Autodesk Inventor part; units mm, degrees
ref_plane "YZ Plane" through (0, 0, 0) normal (1, 0, 0) x (0, 1, 0)
ref_plane "XZ Plane" through (0, 0, 0) normal (0, 1, 0) x (-1, 0, 0)
ref_plane "XY Plane" through (0, 0, 0) normal (0, 0, 1) x (1, 0, 0)
sketch "Sketch1" plane through (0, 0, 0) normal (0, 1, 0) x (-1, 0, 0)
  line L0 (40, 37.5) -> (-40, 37.5)
  line L1 (-40, 37.5) -> (-40, -37.5)
  line L2 (-40, -37.5) -> (40, -37.5)
  line L3 (40, -37.5) -> (40, 37.5)
  line L4 (40, 37.5) -> (-40, -37.5) construction
  line L5 (-40, 37.5) -> (40, -37.5) construction
  point P0 (0, 0)
  dimension "d0" = 80
  dimension "d1" = 75
extrude "Extrusion1" add sketch "Sketch1" along normal blind 3
sketch "Sketch2" plane through (0, 0, 0) normal (0, -1, 0) x (1, 0, 0)
  line L0 (-38, -35.5) -> (38, -35.5)
  line L1 (38, -35.5) -> (38, 35.5)
  line L2 (38, 35.5) -> (-38, 35.5)
  line L3 (-38, 35.5) -> (-38, -35.5)
  line L4 (-38, -35.5) -> (38, 35.5) construction
  line L5 (38, -35.5) -> (-38, 35.5) construction
  line L6 (-40, -37.5) -> (-40, 37.5)
  line L7 (-40, 37.5) -> (40, 37.5)
  line L8 (-40, -37.5) -> (40, -37.5)
  line L9 (40, -37.5) -> (40, 37.5)
  line L10 (40, 37.5) -> (-40, 37.5)
  line L11 (-40, 37.5) -> (-40, -37.5)
  line L12 (-40, -37.5) -> (40, 37.5) construction
  line L13 (40, -37.5) -> (-40, 37.5) construction
  point P0 (0, 0)
  dimension "d4" = 2
  dimension "d5" = 2
extrude "Extrusion2" add sketch "Sketch2" along normal blind 30
sketch "Sketch3" plane through (40, 3, 37.5) normal (1, 0, 0) x (0, 0, -1)
  line L0 (73, -33) -> (2, -33)
  line L1 (12.5, -33) -> (62.5, -33)
  line L2 (62.5, -33) -> (62.5, -24)
  line L3 (62.5, -24) -> (12.5, -24)
  line L4 (12.5, -24) -> (12.5, -33)
  line L5 (75, -33) -> (75, 0)
  point P0 (37.5, -3)
  dimension "d8" = 50
  dimension "d9" = 9
  dimension "d10" = 12.5
extrude "Extrusion3" cut sketch "Sketch3" against normal up to surface (2 mm away)
sketch "Sketch4" plane through (-40, 3, 37.5) normal (0, 0, 1) x (1, 0, 0)
  line L0 (78, -33) -> (2, -33)
  line L1 (2, -33) -> (22, -33)
  line L2 (22, -33) -> (22, -13)
  line L3 (22, -13) -> (2, -13)
  line L4 (2, -13) -> (2, -33)
  line L5 (0, -33) -> (0, 0)
  line L6 (22, -33) -> (28, -33)
  line L7 (28, -33) -> (28, -27)
  line L8 (28, -27) -> (22, -27)
  line L9 (22, -27) -> (22, -33)
  point P0 (40, -3)
  point P1 (22, -27)
  dimension "d13" = 20
  dimension "d14" = 20
  dimension "d15" = 2
  dimension "d16" = 6
  dimension "d17" = 6
extrude "Extrusion4" cut sketch "Sketch4" against normal up to surface (2 mm away)
fillet "Fillet1" radius 2 4 edges at (-38, -10, 36.5) (-18, -10, 36.5) (-12, -24, 36.5) (-18, -24, 36.5)
fillet "Fillet2" radius 2 2 edges at (39, -21, 25) (39, -21, -25)
sketch "Sketch5" plane through (40, 3, -37.5) normal (0, 0, -1) x (-1, 0, 0)
  line L0 (2, -33) -> (78, -33)
  line L1 (78, -33) -> (63, -33)
  line L2 (63, -33) -> (63, -23)
  line L3 (63, -23) -> (78, -23)
  line L4 (78, -23) -> (78, -33)
  line L5 (80, -33) -> (80, 0)
  point P0 (40, -3)
  point P1 (78, -28)
  dimension "d22" = 15
  dimension "d23" = 10
  dimension "d24" = 2
extrude "Extrusion5" cut sketch "Sketch5" against normal up to surface (2 mm away)
fillet "Fillet3" radius 2 3 edges at (-38, -20, -36.5) (-23, -20, -36.5) (-23, -30, -36.5)
sketch "Sketch6" plane through (40, 3, -37.5) normal (0, 0, -1) x (-1, 0, 0)
  circle A0 centre (27, -28) radius 2.25
  line L0 (61, -33) -> (0, -33)
  line L1 (0, -33) -> (0, 0)
  point P0 (40, -3)
  dimension "d28" = 4.5
  dimension "d29" = 5
  dimension "d30" = 27
extrude "Extrusion6" cut sketch "Sketch6" against normal through all
sketch "Sketch7" plane through (-40, 3, -37.5) normal (-1, 0, 0) x (0, 0, 1)
  circle A0 centre (37.5, -28) radius 2.25
  line L0 (75, -33) -> (0, -33)
  line L1 (75, -33) -> (75, 0)
  point P0 (37.5, -3)
  dimension "d33" = 4.5
  dimension "d34" = 5
  dimension "d35" = 37.5
extrude "Extrusion7" cut sketch "Sketch7" against normal up to surface (2 mm away)
fillet "Fillet4" radius 5 4 edges at (-40, 3, 0) (0, 3, 37.5) (0, 3, -37.5) (40, 3, 0)
fillet "Fillet5" radius 5 8 edges at (38.5355, 1.5355, -36.0355) (40, -16, -37.5) (-38.5355, 1.5355, -36.0355) (-40, -16, -37.5) (-38.5355, 1.5355, 36.0355) (-40, -16, 37.5) (38.5355, 1.5355, 36.0355) (40, -16, 37.5)
properties part number "cable_box"
Here's how the part is built. I have some questions about the finished solid (model axes, mm). A direction names the side the tool comes from. Give positions to 0.01 mm unless a question says otherwise; leave off trailing zeros. Order: outer loops, then holes, each group sorted by start corner. A loop starts at its lowest first (then second) coordinate and runs counter-clockwise, first axis right, second up. Notation, with made-up numbers: (-32, -11.75) -> (-8, -11.75) arc R9 cw to (-8, -2.75) -> close; hole circle Ø10 at (-5, 0.5). An arc over 180 degrees is marked (long way). Use CSV: the item, a comma, the result in double quotes. Start each with the question number.
Item 1: Suppose I cut it at D-D (y = -25). Give the number of separate pieces and of enclosed holes in the cut face, and give its area (3 significant figures).
Item 2: If I drill on probe 1 along X at (y, z) = (-6, 19); probe 2 along Z at (x, y) = (-0.5, -18); probe 3 along Y at (x, z) = (17, -19.5), over which ranges is the centre line in solid material (lowest first)? Write a range as [from, to].
Item 3: Thinking about a two-plate mould opening in Y: for faces 4 (the flat face through (9, -15, 35.5)), 5 (the cylindrical face through (13.488, -27.196, 36.486)), 6 (the flat face through (0, 3, 0)), 7 (the cylindrical face through (-39.014, -27.196, -0.488)), which applies, pulls with the +Y half, pulls with the -Y half, needs draft (parallel to the pull), parting line crosses it, or undercut?
Item 4: Suppose I cut it at B-B (y = -7). List the corners of the cut face in (x, z) for me, and give its area (3 significant figures).
Item 5: Suppose I cut it at C-C (z = 0). List the corners of the cut face in (x, y) for me, and give its area (3 significant figures).
Item 6: On a 3-axis mill with a long thin cutter (end or side, diameter ignored), from which of +Z, -Z, +X, -X, +Y, -Y can I reach the whole of each face in a straight line? I mean faces 1 (the cylindrical face through (-37.13, -20.35, -36.23)), 2 (the cylindrical face through (-12.6, -24.57, 36.49)), 3 (the cylindrical face through (38.99, -21.57, -24.4)). Say none if no direction works.
Item 7: Suppose I cut it at A-A (x = 13). List the corners of the cut face in (y, z) for me.
Item 8: I'm going to push flat-ended pins straight in: P1, Ø4, axis at y = -25, z = 0, coming from the +X side (3 decimals); P2, Ø5, axis at x = 13, y = -25, coming from the -Z side; P3, Ø1, axis at y = -29, z = 36.5, coming from the -X side; P4, Ø1.6, axis at x = 39, z = 5.5, coming from the -Y side. Where does each tip first touch, or does it pass through?
Answer block:
1,separate pieces,"6"
1,enclosed holes,"0"
1,area,"376 mm^2"
2,probe 1,"x = [-40, -38], [38, 40]"
2,probe 2,"z = [-37.5, -35.5], [35.5, 37.5]"
2,probe 3,"y = [0, 3]"
3,face 4,"needs draft"
3,face 5,"undercut"
3,face 6,"pulls with the +Y half"
3,face 7,"undercut"
4,outline,"(-40, -32.5) arc R5 ccw to (-35, -37.5) -> (35, -37.5) arc R5 ccw to (40, -32.5) -> (40, 32.5) arc R5 ccw to (35, 37.5) -> (-35, 37.5) arc R5 ccw to (-40, 32.5) -> close; hole (-38, -35.5) -> (38, -35.5) -> (38, 35.5) -> (-38, 35.5) -> close"
4,area,"583 mm^2"
5,outline,"(-40, -30) -> (-38, -30) -> (-38, -27.25) -> (-40, -27.25) -> close; (-40, -22.75) -> (-38, -22.75) -> (-38, 0) -> (38, 0) -> (38, -21) -> (40, -21) -> (40, -2) arc R5 ccw to (35, 3) -> (-35, 3) arc R5 ccw to (-40, -2) -> close"
5,area,"322 mm^2"
6,face 1,"+Z, -Z, -Y"
6,face 2,"+Z, -Y"
6,face 3,"+X, -Y"
7,outline,"(-30, -37.5) -> (-27.25, -37.5) -> (-27.25, -35.5) -> (-30, -35.5) -> close; (-30, 35.5) -> (-27.25, 35.5) -> (-27.25, 37.5) -> (-30, 37.5) -> close; (-22.75, -37.5) -> (-2, -37.5) arc R5 ccw to (3, -32.5) -> (3, 32.5) arc R5 ccw to (-2, 37.5) -> (-22.75, 37.5) -> (-22.75, 35.5) -> (0, 35.5) -> (0, -35.5) -> (-22.75, -35.5) -> close"
8,P1,"passes through"
8,P2,"stops at z = -37.5"
8,P3,"stops at x = -38.57"
8,P4,"stops at y = -21"
